Job drawing, mm, ordinate dimensions from the low corner. One solid piece. A direction names the side the tool comes from. Give positions to 0.01 mm unless a question says otherwise; leave off trailing zeros. Loops run counter-clockwise (first coordinate to the right, second up) from the corner with the lowest first, then second, coordinate; pieces in that order, holes last. Notation, with made-up numbers: M -7.5,-30 L 27.5,-30 A18 cw 27.5,-23 Z; hole C 14.25,39.25 d5. An arc over 180 degrees is marked long. Answer as CSV lines item,"result".
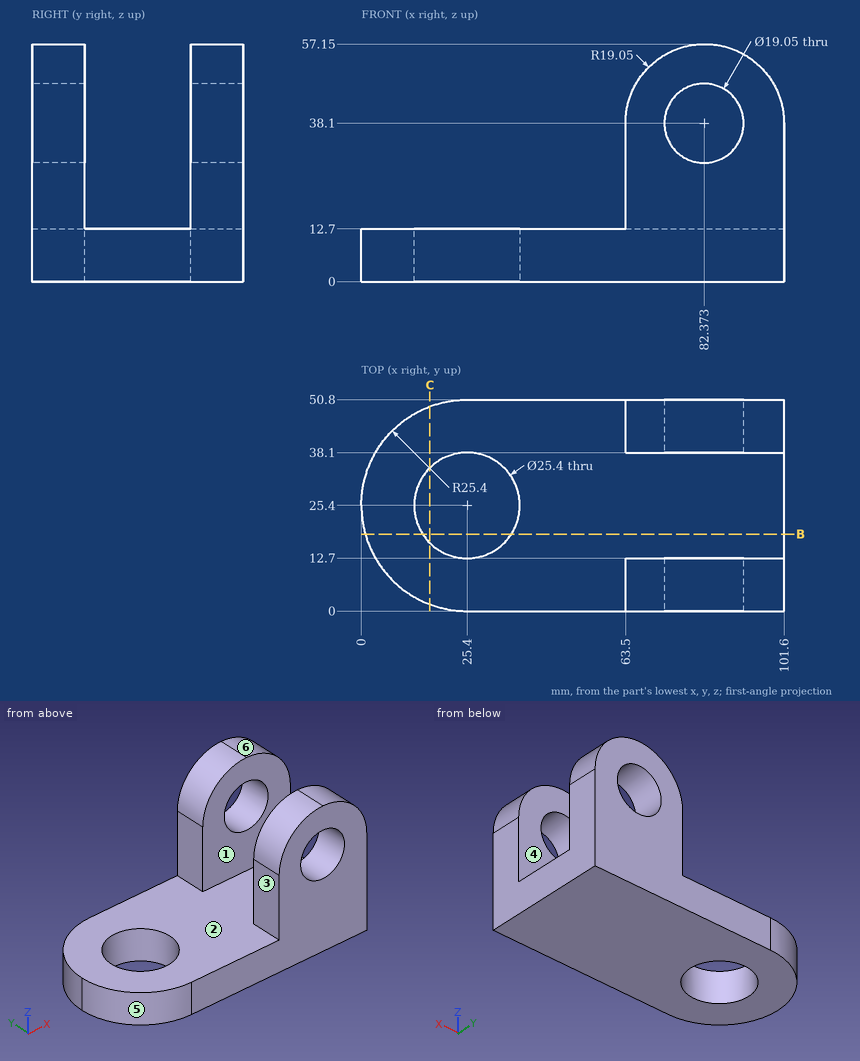
1) Mould opens along Y. For the marked faces 4, 5 and 6 say: +Y half, -Y half, draft (parallel to the pull), parting line (faces both ways), or undercut.
Answer below:
face 4,"undercut"
face 5,"-Y half"
face 6,"draft"
2) Flat gauge pins, fed straight in: pin 1 (11.5 mm diameter, centred on x = 82.37, z = 38.1, fed in from +Y); pin 2 (14 mm diameter, centred on y = 9.5, z = 30, fed in from -X); pin 3 (2 mm diameter, centred on x = 84.5, y = 35.5, fed in from +Z); pin 4 (2 mm diameter, centred on x = 32, y = 9, fed in from -Z). Where does each tip first touch, or does it go through?
Answer below:
pin 1,"passes through"
pin 2,"stops at x = 63.5"
pin 3,"stops at z = 12.7"
pin 4,"stops at z = 0"
3) Which spindle directions (+Z, -Z, +X, -X, +Y, -Y) get a long thin tool onto all of the face, cutting with end or side? Do the marked faces 1, 2 and 3. Say none if no direction does.
Answer below:
face 1,"+Z, +X, -X"
face 2,"+Z, -X"
face 3,"+Z, -X, +Y, -Y"
4) Band-saw the part on C-C on x = 16.5. Give the cut face in (y, z).
Answer below:
outline,"M 1.61,0 L 16.34,0 L 16.34,12.7 L 1.61,12.7 Z; M 34.46,0 L 49.19,0 L 49.19,12.7 L 34.46,12.7 Z"
5) Band-saw the part on B-B on y = 18.5. Give the cut face in (x, z) (1 decimal), and give its area (3 significant figures).
Answer below:
outline,"M 1,0 L 14.7,0 L 14.7,12.7 L 1,12.7 Z; M 36.1,0 L 101.6,0 L 101.6,12.7 L 36.1,12.7 Z"
area,"1,010 mm^2"
6) Drill centre lines: line 1 (Y direction, x = 91, z = 51); line 2 (X direction, y = 9, z = 38); line 3 (Y direction, x = 34, z = 12) (1 decimal). Where is each one in solid material? Low to high. Write a range as from..to.
Answer below:
line 1,"y = 0..12.7, 38.1..50.8"
line 2,"x = 63.5..72.85, 91.9..101.6"
line 3,"y = 0..16.1, 34.7..50.8"
